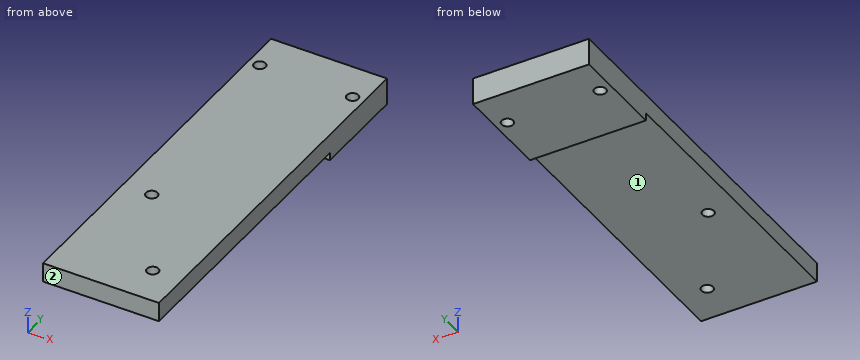
from build123d import *

# Parameters (mm, degrees)
SALIENTE_EXTRUIR1_START = 2
SALIENTE_EXTRUIR1_DEPTH = 5
CROQUIS2_W              = 30
CROQUIS2_H              = 25
SALIENTE_EXTRUIR2_DEPTH = 2
CROQUIS3_R              = 1.5
CORTAR_EXTRUIR1_DEPTH   = 10
CROQUIS4_R              = 1.500036904
CROQUIS4_R_2            = 1.5
CORTAR_EXTRUIR2_DEPTH   = 10


with BuildPart() as part:
    # Croquis1 → Saliente-Extruir1 (new body)
    with BuildSketch(Plane.XY.offset(SALIENTE_EXTRUIR1_START)):
        Polygon((65.454041039, -1015), (65.454041039, -1005), (95.454041039, -1005), (95.454041039, -1015), (95.454041039, -1105), (65.454041039, -1105), align=None)
    extrude(amount=SALIENTE_EXTRUIR1_DEPTH)

    # Croquis2 → Saliente-Extruir2 (add)
    with BuildSketch(Plane(origin=(0, 0, 2), x_dir=(-1, 0, 0), z_dir=(0, 0, -1))):
        with Locations((-80.454041039, -1017.5)):
            Rectangle(CROQUIS2_W, CROQUIS2_H)
    extrude(amount=SALIENTE_EXTRUIR2_DEPTH)

    # Croquis3 → Cortar-Extruir1 (cut)
    with BuildSketch(Plane(origin=(0, 0, 2), x_dir=(-1, 0, 0), z_dir=(0, 0, -1))):
        with Locations((-72.954041039, -1070)):
            Circle(CROQUIS3_R)
        with Locations((-87.954041039, -1095)):
            Circle(CROQUIS3_R)
    extrude(amount=-CORTAR_EXTRUIR1_DEPTH, mode=Mode.SUBTRACT)

    # Croquis4 → Cortar-Extruir2 (cut)
    with BuildSketch(Plane(origin=(0, 0, 0), x_dir=(-1, 0, 0), z_dir=(0, 0, -1))):
        with Locations((-92.454041038, -1014.999963096)):
            Circle(CROQUIS4_R)
        with Locations((-68.454041039, -1015)):
            Circle(CROQUIS4_R_2)
    extrude(amount=-CORTAR_EXTRUIR2_DEPTH, mode=Mode.SUBTRACT)


solid = part.part
CAD build for the part. Positions are in the model's coordinates, mm. Face numbers are marked on the shaded views. A direction names the side the tool comes from. Give positions to 0.01 mm unless a question says otherwise; leave off trailing zeros. Order: outer loops, then holes, each group sorted by start corner. A loop starts at its lowest first (then second) coordinate and runs counter-clockwise, first axis right, second up. Notation, with made-up numbers: (38, 58) - (73, 58) arc R20 ccw to (73, 82) - close; hole circle Ø10 at (50.5, 75). An arc over 180 degrees is marked (long way). Write each question's results on one line, items separated by ' | '.
1. Saw through at C-C on x = 78.5. List the corners of the cut face in (y, z).
Calculated:
outline: (-1105, 2) - (-1030, 2) - (-1030, 0) - (-1005, 0) - (-1005, 7) - (-1105, 7) - close
2. Saw through at B-B on x = 73.5. List the corners of the cut face in (y, z).
Calculated:
outline: (-1105, 2) - (-1071.4, 2) - (-1071.4, 7) - (-1105, 7) - close; (-1068.6, 2) - (-1030, 2) - (-1030, 0) - (-1005, 0) - (-1005, 7) - (-1068.6, 7) - close
3. Pin check, flat tips, straight feed: pin 1 (1 mm diameter, centred on x = 74, z = 0.5, fed in from -Y); pin 2 (5 mm diameter, centred on x = 72.95, y = -1070, fed in from -Z). Stop position of each tip, or through.
Calculated:
pin 1: stops at y = -1030 | pin 2: stops at z = 2
4. Saw through at D-D on y = -1037.5. List the corners of the cut face in (x, z).
Calculated:
outline: (65.45, 2) - (95.45, 2) - (95.45, 7) - (65.45, 7) - close
5. Probe L1, parallel to X at y = -1015, z = 3.75; L2, parallel to X at y = -1070, z = 3.7; L3, parallel to Y at x = 88, z = 4.5. List the from-to ranges inside material, lowest first. Write a range as from..to.
Calculated:
L1: x = 65.45..66.95, 69.95..90.95, 93.95..95.45 | L2: x = 65.45..71.45, 74.45..95.45 | L3: y = -1105..-1096.5, -1093.5..-1005
6. 3-axis set-ups, long thin cutter, end or side, ignore diameter. For the marked faces 1 and 2: which of +Z, -Z, +X, -X, +Y, -Y reach the whole face in a straight line?
Calculated:
face 1: -Z, +X, -X, -Y | face 2: +Z, -Z, +X, -X, -Y
7. Saw through at A-A on y = -1095. List the corners of the cut face in (x, z).
Calculated:
outline: (65.45, 2) - (86.45, 2) - (86.45, 7) - (65.45, 7) - close; (89.45, 2) - (95.45, 2) - (95.45, 7) - (89.45, 7) - close
